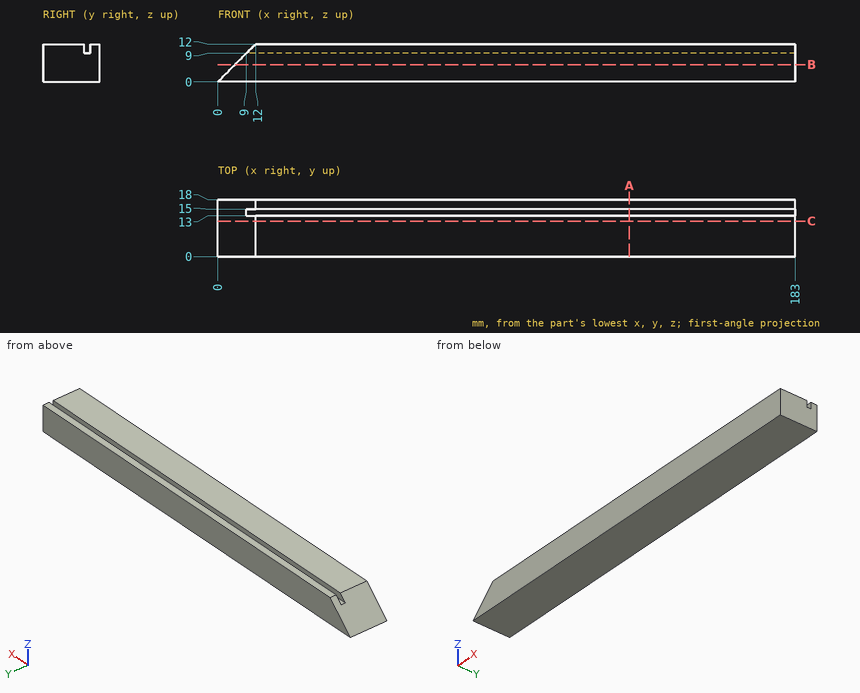
Here's the drawing with two shaded views (mm, measured from the low corner). I have some questions. Coordinates: 2 decimals unless noted, no trailing zeros. Order: outer loops, then holes, each group sorted by start corner. A loop starts at its lowest first (then second) coordinate and runs counter-clockwise, first axis right, second up. Notation, with made-up numbers: M 34,40 L 45,40 A22 ccw 45,65 Z; hole C 69,0 d2. An arc over 180 degrees is marked long. Answer as CSV lines item,"result".
Item 1: Imagine slicing it at A-A on x = 130.5. Write out the boundary of the cut face in (y, z), plus the area to 3 significant figures.
Results found:
outline,"M 0,0 L 18,0 L 18,12 L 15,12 L 15,9 L 13,9 L 13,12 L 0,12 Z"
area,"210 mm2"
Item 2: Imagine slicing it at C-C on y = 11.25. Write out the boundary of the cut face in (x, z), plus the area to 3 significant figures.
Results found:
outline,"M 0,0 L 183,0 L 183,12 L 12,12 Z"
area,"2,120 mm2"
Item 3: If I drill on line 1 (Y direction, x = 126, z = 9.5); line 2 (X direction, y = 9.25, z = 4.5); line 3 (X direction, y = 16.5, z = 5), over which ranges is the centre line in solid material (lowest first)?
Results found:
line 1,"0 to 13, 15 to 18"
line 2,"4.5 to 183"
line 3,"5 to 183"
Item 4: Imagine slicing it at B-B on z = 5.5. Write out the boundary of the cut face in (x, y).
Results found:
outline,"M 5.5,0 L 183,0 L 183,18 L 5.5,18 Z"
Item 5: For pin 1 (4 mm diameter, centred on y = 5, z = 9, fed in from -X); pin 2 (2 mm diameter, centred on y = 8.5, z = 2, fed in from -X); pin 3 (4 mm diameter, centred on y = 12.5, z = 5.5, fed in from -X), each with a flat end and sliding along its axis, tell me the tip position at first contact or that it passes through.
Results found:
pin 1,"x = 7"
pin 2,"x = 1"
pin 3,"x = 3.5"
